Check sheet for the modelled part. Datum: model origin and axes. Units: mm. Face numbers are marked on the shaded views. A direction names the side the tool comes from. Give positions to 0.01 mm unless a question says otherwise; leave off trailing zeros. Write each loop counter-clockwise with the first axis right and the second up, starting at its lowest first coordinate (ties: lowest second). Pieces come first, ordered by that corner, then holes. Notation, with made-up numbers: M 67.5,39.5 L 107.5,39.5 A21 cw 107.5,69.5 Z; hole C 40.25,79.25 d9. An arc over 180 degrees is marked long. Write each question's results on one line, items separated by ' | '. Start each with the question number.
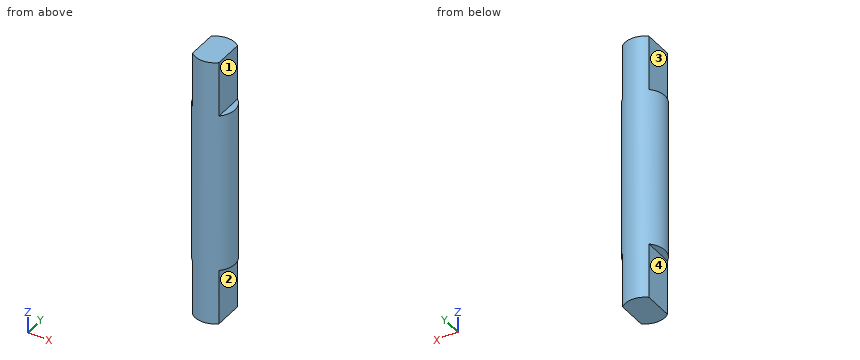
from build123d import *

# Parameters (mm, degrees)
CROQUIS1_R              = 2.7
SALIENTE_EXTRUIR1_DEPTH = 36.7
CORTAR_EXTRUIR1_DEPTH   = 7.5
CORTAR_EXTRUIR2_START   = -7.5
CORTAR_EXTRUIR2_DEPTH   = 7.5


with BuildPart() as part:
    # Croquis1 → Saliente-Extruir1 (new body)
    with BuildSketch(Plane.XY):
        Circle(CROQUIS1_R)
    extrude(amount=SALIENTE_EXTRUIR1_DEPTH)

    # Croquis2 → Cortar-Extruir1 (cut)
    with BuildSketch(Plane(origin=(0, 0, 0), x_dir=(-1, 0, 0), z_dir=(0, 0, -1))):
        with BuildLine():
            ThreePointArc((-1.8, 2.01246118), (-2.7, 0), (-1.8, -2.01246118))
            Line((-1.8, -2.01246118), (-1.8, 2.01246118))
        make_face()
        with BuildLine():
            Line((1.8, 2.01246118), (1.8, -2.01246118))
            ThreePointArc((1.8, -2.01246118), (2.464751509, -1.102270384), (2.7, 0))
            ThreePointArc((2.7, 0), (2.464751509, 1.102270384), (1.8, 2.01246118))
        make_face()
    extrude(amount=-CORTAR_EXTRUIR1_DEPTH, mode=Mode.SUBTRACT)

    # Croquis3 → Cortar-Extruir2 (cut)
    with BuildSketch(Plane.XY.offset(36.7).offset(CORTAR_EXTRUIR2_START)):
        with BuildLine():
            Line((1.8, 2.01246118), (1.8, -2.01246118))
            ThreePointArc((1.8, -2.01246118), (2.464751509, -1.102270384), (2.7, 0))
            ThreePointArc((2.7, 0), (2.464751509, 1.102270384), (1.8, 2.01246118))
        make_face()
        with BuildLine():
            ThreePointArc((-1.8, 2.01246118), (-2.7, 0), (-1.8, -2.01246118))
            Line((-1.8, -2.01246118), (-1.8, 2.01246118))
        make_face()
    extrude(amount=CORTAR_EXTRUIR2_DEPTH, mode=Mode.SUBTRACT)


solid = part.part
Q1. Tool access check on the marked faces 1, 2, 3 and 4. Record the directions out of +Z, -Z, +X, -X, +Y, -Y that give a thin tool (end or side, any length) a straight path to the whole face; none if there is none.
Q2. Depth check by flat-ended pin: pin 1 Ø3 at (y, z) = (0, 34.5) entering from +X; pin 2 Ø0.7 at (x, y) = (2.5, 1) entering from +Z; pin 3 Ø2 at (y, z) = (0, 33.5) entering from -X. Enter the tip coordinate at first touch or a pass-through.
Q3. Section check A-A on y = 0. Record the boundary of the cut face in (x, z), plus the area to 3 significant figures.
Q4. Section check C-C on y = 1.35. Record the boundary of the cut face in (x, z).
Q5. Section check B-B on z = 30.5. Record the boundary of the cut face in (x, y).
Q6. Scan lines: L1, parallel to Z at x = -2.15, y = 1.15; L2, parallel to X at y = -0.55, z = 2; L3, parallel to X at y = 1.9, z = 16.5. Record each from-to range of solid material in increasing order.
Q7. Section check D-D on x = 0.6. Record the boundary of the cut face in (y, z), plus the area to 3 significant figures.
Check result:
1) face 1: +Z, +X, +Y, -Y | face 2: -Z, +X, +Y, -Y | face 3: +Z, -X, +Y, -Y | face 4: -Z, -X, +Y, -Y
2) pin 1: x = 1.8 | pin 2: z = 29.2 | pin 3: x = -1.8
3) outline: M -2.7,7.5 L -1.8,7.5 L -1.8,0 L 1.8,0 L 1.8,7.5 L 2.7,7.5 L 2.7,29.2 L 1.8,29.2 L 1.8,36.7 L -1.8,36.7 L -1.8,29.2 L -2.7,29.2 Z | area: 171 mm^2
4) outline: M -2.34,7.5 L -1.8,7.5 L -1.8,0 L 1.8,0 L 1.8,7.5 L 2.34,7.5 L 2.34,29.2 L 1.8,29.2 L 1.8,36.7 L -1.8,36.7 L -1.8,29.2 L -2.34,29.2 Z
5) outline: M -1.8,-2.01 A2.7 ccw 1.8,-2.01 L 1.8,2.01 A2.7 ccw -1.8,2.01 Z
6) L1: 7.5 to 29.2 | L2: -1.8 to 1.8 | L3: -1.92 to 1.92
7) outline: M -2.63,0 L 2.63,0 L 2.63,36.7 L -2.63,36.7 Z | area: 193 mm^2
